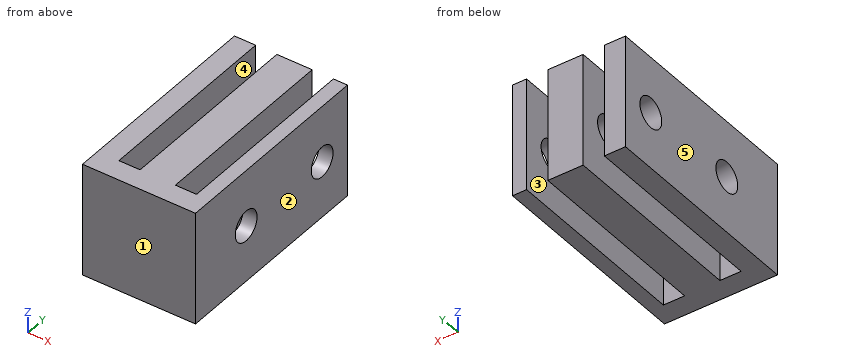
from build123d import *

# Parameters (mm, degrees)
SKETCH1_W           = 16
SKETCH1_H           = 16
BOSS_EXTRUDE1_DEPTH = 30
SKETCH2_W           = 3
SKETCH2_H           = 27
CUT_EXTRUDE1_DEPTH  = 17
SKETCH3_R           = 2.15
CUT_EXTRUDE2_DEPTH  = 17


with BuildPart() as part:
    # Sketch1 → Boss-Extrude1 (new body)
    with BuildSketch(Plane(origin=(0, 0, 0), x_dir=(1, 0, 0), z_dir=(0, 1, 0))):
        with Locations((8, 8)):
            Rectangle(SKETCH1_W, SKETCH1_H)
    extrude(amount=BOSS_EXTRUDE1_DEPTH)

    # Sketch2 → Cut-Extrude1 (cut, through all)
    with BuildSketch(Plane.XY):
        with Locations((4.5, 16.5)):
            Rectangle(SKETCH2_W, SKETCH2_H)
        with Locations((12.5, 16.5)):
            Rectangle(SKETCH2_W, SKETCH2_H)
    extrude(amount=-CUT_EXTRUDE1_DEPTH, mode=Mode.SUBTRACT)

    # Sketch3 → Cut-Extrude2 (cut, through all)
    with BuildSketch(Plane.ZY):
        with Locations((-8, 25)):
            Circle(SKETCH3_R)
        with Locations((-8, 10)):
            Circle(SKETCH3_R)
    extrude(amount=-CUT_EXTRUDE2_DEPTH, mode=Mode.SUBTRACT)


solid = part.part
Design review of the part built by this model. Coordinates are the model's own, in mm. Face numbers are marked on the shaded views. A direction names the side the tool comes from. Give positions to 0.01 mm unless a question says otherwise; leave off trailing zeros. Order: outer loops, then holes, each group sorted by start corner. A loop starts at its lowest first (then second) coordinate and runs counter-clockwise, first axis right, second up. Notation, with made-up numbers: (-13, 9) - (39, 9) arc R23 cw to (39, 29) - close; hole circle Ø7 at (20, 13). An arc over 180 degrees is marked (long way). Write item = value, one per line. Start each with the question number.
Q1. To check wall thickness, follow L1, parallel to X at y = 18, z = -13; L2, parallel to Y at x = 7.7, z = -8; L3, parallel to Y at x = 4, z = -2. State the ranges of each line that lie inside material, in increasing order. Write a range as from..to.
Q2. We need section A-A on y = 25. State the section outline as (x, z) points.
Q3. We need section B-B on x = 8.5. State the section outline as (y, z) points.
Q4. Tool access review of the marked faces 4 and 5: name each direction out of +Z, -Z, +X, -X, +Y, -Y from which nothing blocks a thin tool from reaching the whole face with its end or side.
Q5. We need section D-D on z = -2.5. State the section outline as (x, y) points.
Q6. Mouldability with a two-part tool opening along X and no side actions: class the marked faces 1, 2 and 3 as released by +X, released by -X, zero draft, split by the parting line, or undercut.
Q7. Clearance check with flat-ended pins moving along their axes: pin 1 Ø4 at (y, z) = (10, -8) entering from +X; pin 2 Ø0.9 at (x, z) = (4.5, -5) entering from +Y. State where each tip first meets the part, or that it passes through.
Q8. We need section C-C on y = 6.25. State the section outline as (x, z) points, plus the area to 3 significant figures.
Working result:
q1.L1 = 0..3, 6..11, 14..16
q1.L2 = 0..7.85, 12.15..22.85, 27.15..30
q1.L3 = 0..3
q2.outline = (0, -16) - (3, -16) - (3, -10.15) - (0, -10.15) - close; (0, -5.85) - (3, -5.85) - (3, 0) - (0, 0) - close; (6, -16) - (11, -16) - (11, -10.15) - (6, -10.15) - close; (6, -5.85) - (11, -5.85) - (11, 0) - (6, 0) - close; (14, -16) - (16, -16) - (16, -10.15) - (14, -10.15) - close; (14, -5.85) - (16, -5.85) - (16, 0) - (14, 0) - close
q3.outline = (0, -16) - (30, -16) - (30, 0) - (0, 0) - close; hole circle Ø4.3 at (10, -8); hole circle Ø4.3 at (25, -8)
q4.face_4 = +Z, -Z, +Y
q4.face_5 = +Z, -Z, -X, +Y, -Y
q5.outline = (0, 0) - (16, 0) - (16, 30) - (14, 30) - (14, 3) - (11, 3) - (11, 30) - (6, 30) - (6, 3) - (3, 3) - (3, 30) - (0, 30) - close
q6.face_1 = zero draft
q6.face_2 = released by +X
q6.face_3 = undercut
q7.pin_1 = through
q7.pin_2 = 3
q8.outline = (0, -16) - (3, -16) - (3, 0) - (0, 0) - close; (6, -16) - (11, -16) - (11, 0) - (6, 0) - close; (14, -16) - (16, -16) - (16, 0) - (14, 0) - close
q8.area = 160 mm²
